Work out the finished part from the listing and answer in its coordinate system (mm). Give positions to 0.01 mm unless a question says otherwise; leave off trailing zeros. Write each loop counter-clockwise with the first axis right and the second up, starting at its lowest first coordinate (ties: lowest second). Pieces come first, ordered by that corner, then holes.
1) Straight lines are drawn through the part: probe 1 along Y at (x, z) = (-30, 1.2); probe 2 along Y at (x, z) = (-27, 1.05); probe 3 along X at (y, z) = (8, 0.75). For each, find the intervals that lie inside material, in ascending order.
2) Find section A-A (z = 0.95). Determine the outline of the cut face in (x, y).
3) Find section D-D (x = -54). Determine the outline of the cut face in (y, z).
4) Find section C-C (y = 9.5). Determine the outline of the cut face in (x, z).
5) Find section B-B (x = -31.5). Determine the outline of the cut face in (y, z), plus the area to 3 significant figures.
Autodesk Inventor part; units mm, degrees
ref_plane "YZ Plane" through (0, 0, 0) normal (1, 0, 0) x (0, 1, 0)
ref_plane "XZ Plane" through (0, 0, 0) normal (0, 1, 0) x (-1, 0, 0)
ref_plane "XY Plane" through (0, 0, 0) normal (0, 0, 1) x (1, 0, 0)
sketch "Sketch1" plane through (0, 0, 0) normal (0, 0, 1) x (1, 0, 0)
  line L0 (-25, 0) -> (-35, 0)
  line L1 (-60, 25) -> (-60, 60)
  line L2 (-60, 60) -> (0, 60)
  line L3 (0, 60) -> (0, 25)
  arc A0 (-25, 0) -> (0, 25) centre (-25, 25) ccw
  arc A1 (-60, 25) -> (-35, 0) centre (-35, 25) ccw
  point P0 (0, 0)
  point P1 (-60, 0)
  dimension "d0" = 60
  dimension "d1" = 60
  dimension "d9" = 25
extrude "Extrusion1" add sketch "Sketch1" along normal blind 1.5
sketch "Sketch2" plane through (0, 0, 1.5) normal (0, 0, 1) x (1, 0, 0)
  line L0 (0, 0) -> (-30, 0)
  line L1 (-35, 0) -> (0, 0)
  line L2 (-30, 3.5) -> (-30, 8)
  circle A0 centre (-30, 8) radius 4.5
  point P0 (-60, 0)
  dimension "d6" = 9
  dimension "d4" = 30
  dimension "d5" = 8
extrude "Extrusion2" cut sketch "Sketch2" against normal blind 1.5
properties part number "clamp"
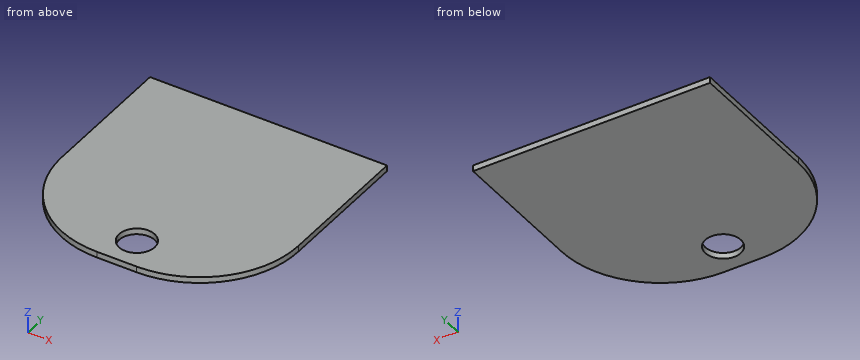
Results:
1. probe 1: y = 0 to 3.5, 12.5 to 60
1. probe 2: y = 0 to 4.65, 11.35 to 60
1. probe 3: x = -53.33 to -34.5, -25.5 to -6.67
2. outline: (-60, 25) arc R25 ccw to (-35, 0) - (-25, 0) arc R25 ccw to (0, 25) - (0, 60) - (-60, 60) - close; hole circle Ø9 at (-30, 8)
3. outline: (8.75, 0) - (60, 0) - (60, 1.5) - (8.75, 1.5) - close
4. outline: (-54.62, 0) - (-34.24, 0) - (-34.24, 1.5) - (-54.62, 1.5) - close; (-25.76, 0) - (-5.38, 0) - (-5.38, 1.5) - (-25.76, 1.5) - close
5. outline: (0, 0) - (3.76, 0) - (3.76, 1.5) - (0, 1.5) - close; (12.24, 0) - (60, 0) - (60, 1.5) - (12.24, 1.5) - close
5. area: 77.3 mm2
